```python
from build123d import *

# Parameters (mm, degrees)
CROQUIS1_R                   = 115.062
CROQUIS1_R_2                 = 31.75
SALIENTE_EXTRUIR1_DEPTH      = 50
CORPS_D_PLACER_COPIER1_ANGLE = 90


with BuildPart() as part:
    # Croquis1 → Saliente-Extruir1 (new body)
    with BuildSketch(Plane.XY):
        with BuildLine():
            Line((-72.263, -175.395747529), (-72.263, -249.055747529))
            Line((-72.263, -249.055747529), (-72.263, -250.444))
            ThreePointArc((-72.263, -250.444), (-74.494846327, -255.832153673), (-79.883, -258.064))
            Line((-79.883, -258.064), (-80.137, -258.064))
            Line((-80.137, -258.064), (-80.137, -418.338))
            Line((-80.137, -418.338), (80.137, -418.338))
            Line((80.137, -418.338), (80.137, -258.064))
            Line((80.137, -258.064), (79.883, -258.064))
            ThreePointArc((79.883, -258.064), (74.494846327, -255.832153673), (72.263, -250.444))
            Line((72.263, -250.444), (72.263, -249.055747529))
            Line((72.263, -249.055747529), (72.263, -175.395747529))
            Line((72.263, -175.395747529), (137.414, -33.979836109))
            Line((137.414, -33.979836109), (137.414, 171.760163891))
            ThreePointArc((137.414, 171.760163891), (0, 219.964), (-137.414, 171.760163891))
            Line((-137.414, 171.760163891), (-137.414, -33.979836109))
            Line((-137.414, -33.979836109), (-72.263, -175.395747529))
        make_face()
        Circle(CROQUIS1_R, mode=Mode.SUBTRACT)
        with Locations((0, -338.201)):
            Circle(CROQUIS1_R_2, mode=Mode.SUBTRACT)
    extrude(amount=SALIENTE_EXTRUIR1_DEPTH)


with BuildPart() as part_1:
    # Corps-Déplacer/Copier1: moved
    add(part.part.rotate(Axis((0, 0, 0), (0, 0, 1)), CORPS_D_PLACER_COPIER1_ANGLE))


solid = part_1.part
```
Read the model definition and answer for the solid it produces. Units are mm, in the model's axes. A direction names the side the tool comes from. Give positions to 0.01 mm unless a question says otherwise; leave off trailing zeros. Write each loop counter-clockwise with the first axis right and the second up, starting at its lowest first coordinate (ties: lowest second). Pieces come first, ordered by that corner, then holes. Notation, with made-up numbers: (-6.5, -6.5) -> (5.5, -6.5) arc R10 ccw to (5.5, 10.5) -> close; hole circle Ø9 at (20, 41). An arc over 180 degrees is marked (long way). Answer in a Markdown table with one row per item.
1) Each of these flat-tipped pins is pushed along its axis until it touches: pin 1 Ø12 at (x, z) = (88, 36) entering from +Y; pin 2 Ø4 at (y, z) = (67.5, 17.5) entering from -X; pin 3 Ø25 at (x, z) = (371.5, 28.5) entering from -Y. Where does it stop, or does it pass through?
Results list:
| item | result |
|---|---|
| pin 1 | y = 115.29 |
| pin 2 | x = -209.99 |
| pin 3 | y = -80.14 |
2) Section C-C on z = 7 is taken. Give the vertices of the cut face in (x, y), plus the area to 3 significant figures.
Results list:
| item | result |
|---|---|
| outline | (-171.76, -137.41) -> (33.98, -137.41) -> (175.4, -72.26) -> (250.44, -72.26) arc R7.62 cw to (258.06, -79.88) -> (258.06, -80.14) -> (418.34, -80.14) -> (418.34, 80.14) -> (258.06, 80.14) -> (258.06, 79.88) arc R7.62 cw to (250.44, 72.26) -> (175.4, 72.26) -> (33.98, 137.41) -> (-171.76, 137.41) arc R219.96 ccw to start; hole circle Ø230.12 at (0, 0); hole circle Ø63.5 at (338.2, 0) |
| area | 88,100 mm^2 |
3) Section A-A on x = 0 is taken. Give the vertices of the cut face in (y, z).
Results list:
| item | result |
|---|---|
| outline | (-137.41, 0) -> (-115.06, 0) -> (-115.06, 50) -> (-137.41, 50) -> close; (115.06, 0) -> (137.41, 0) -> (137.41, 50) -> (115.06, 50) -> close |
4) Section B-B on y = 0 is taken. Give the vertices of the cut face in (x, z), plus the area to 3 significant figures.
Results list:
| item | result |
|---|---|
| outline | (-219.96, 0) -> (-115.06, 0) -> (-115.06, 50) -> (-219.96, 50) -> close; (115.06, 0) -> (306.45, 0) -> (306.45, 50) -> (115.06, 50) -> close; (369.95, 0) -> (418.34, 0) -> (418.34, 50) -> (369.95, 50) -> close |
| area | 17,200 mm^2 |
5) Section D-D on y = 91.5 is taken. Give the vertices of the cut face in (x, z), plus the area to 3 significant figures.
Results list:
| item | result |
|---|---|
| outline | (-200.03, 0) -> (-69.76, 0) -> (-69.76, 50) -> (-200.03, 50) -> close; (69.76, 0) -> (133.64, 0) -> (133.64, 50) -> (69.76, 50) -> close |
| area | 9,710 mm^2 |
6) Straight lines are drawn through the part: line 1 (X direction, y = 0, z = 36); line 2 (Y direction, x = 382.5, z = 46.5); line 3 (Y direction, x = -0.5, z = 20). For each, find the intervals that lie inside material, in ascending order. Write a range as [from, to].
Results list:
| item | result |
|---|---|
| line 1 | [-219.96, -115.06], [115.06, 306.45], [369.95, 418.34] |
| line 2 | [-80.14, 80.14] |
| line 3 | [-137.41, -115.06], [115.06, 137.41] |
7) A tool of negligible diameter and unlimited length cuts with its end or side. For faces 1 (the flat face through (212, -72.263, 25)), 2 (the flat face through (339, 80.137, 25)), 3 (the flat face through (337, -80.137, 25)), from which of +Z, -Z, +X, -X, +Y, -Y can it reach the whole face along a straight path? Write none if from no direction.
Results list:
| item | result |
|---|---|
| face 1 | +Z, -Z, -Y |
| face 2 | +Z, -Z, +X, +Y |
| face 3 | +Z, -Z, +X, -Y |
